CAD build for the part. Positions are in the model's coordinates, mm. A direction names the side the tool comes from. Give positions to 0.01 mm unless a question says otherwise; leave off trailing zeros. Loops run counter-clockwise (first coordinate to the right, second up) from the corner with the lowest first, then second, coordinate; pieces in that order, holes last. Notation, with made-up numbers: M 9.5,-39 L 45.5,-39 A23 cw 45.5,-23 Z; hole C 84.25,30.25 d11. An arc over 180 degrees is marked long. One line per question, with ' | ' between items.
```python
from build123d import *

# Parameters (mm, degrees)
BOSS_EXTRUDE1_DEPTH = 8
CUT_EXTRUDE1_DEPTH  = 1
SKETCH4_W           = 16
SKETCH4_H           = 7
CUT_EXTRUDE2_DEPTH  = 1
SHELL3_START        = 2
SHELL3_DEPTH        = 5.5
SHELL3_START_2      = 0.5
SHELL3_2_DEPTH      = 1.5
SHELL3_START_3      = 1.5
SHELL3_3_OUTLINE_W  = 17
SHELL3_3_OUTLINE_H  = 8
SHELL3_3_DEPTH      = 0.5


# Read off the part's stored shape, not the designer's step: Shell3
with BuildPart() as part:
    # Sketch2 → Boss-Extrude1 (new body)
    with BuildSketch(Plane(origin=(0, 0, 0), x_dir=(1, 0, 0), z_dir=(0, 1, 0))):
        with BuildLine():
            Line((-15, -10), (15, -10))
            ThreePointArc((15, -10), (25, 0), (15, 10))
            Line((15, 10), (-15, 10))
            ThreePointArc((-15, 10), (-25, 0), (-15, -10))
        make_face()
    extrude(amount=BOSS_EXTRUDE1_DEPTH)

    # Sketch3 → Cut-Extrude1 (cut)
    with BuildSketch(Plane.XZ):
        with BuildLine():
            Line((-5, 5), (5, 5))
            ThreePointArc((5, 5), (10, 0), (5, -5))
            Line((5, -5), (-5, -5))
            ThreePointArc((-5, -5), (-10, 0), (-5, 5))
        make_face()
    extrude(amount=-CUT_EXTRUDE1_DEPTH, mode=Mode.SUBTRACT)

    # Sketch4 → Cut-Extrude2 (cut)
    with BuildSketch(Plane.XZ.offset(-1)):
        Rectangle(SKETCH4_W, SKETCH4_H)
    extrude(amount=-CUT_EXTRUDE2_DEPTH, mode=Mode.SUBTRACT)

    # Shell3 outline → Shell3 (cut)
    with BuildSketch(Plane(origin=(0, 0, 0), x_dir=(1, 0, 0), z_dir=(0, 1, 0)).offset(SHELL3_START)):
        with BuildLine():
            Line((15, 9.5), (15, 10))
            Line((15, 10), (-15, 10))
            Line((-15, 10), (-15, 9.5))
            ThreePointArc((-15, 9.5), (-24.5, 0), (-15, -9.5))
            Line((-15, -9.5), (15, -9.5))
            ThreePointArc((15, -9.5), (24.5, 0), (15, 9.5))
        make_face()
    extrude(amount=SHELL3_DEPTH, mode=Mode.SUBTRACT)

    # Shell3 2 outline → Shell3 2 (cut)
    with BuildSketch(Plane(origin=(0, 0, 0), x_dir=(1, 0, 0), z_dir=(0, 1, 0)).offset(SHELL3_START_2)):
        with BuildLine():
            Line((15, 9.5), (15, 10))
            Line((15, 10), (-15, 10))
            Line((-15, 10), (-15, 9.5))
            ThreePointArc((-15, 9.5), (-24.5, 0), (-15, -9.5))
            Line((-15, -9.5), (15, -9.5))
            ThreePointArc((15, -9.5), (24.5, 0), (15, 9.5))
        make_face()
        with BuildLine():
            Line((5, -5.5), (-5, -5.5))
            ThreePointArc((-5, -5.5), (-10.5, 0), (-5, 5.5))
            Line((-5, 5.5), (5, 5.5))
            ThreePointArc((5, 5.5), (10.5, 0), (5, -5.5))
        make_face(mode=Mode.SUBTRACT)
    extrude(amount=SHELL3_2_DEPTH, mode=Mode.SUBTRACT)

    # Shell3 3 outline → Shell3 3 (cut)
    with BuildSketch(Plane(origin=(0, 0, 0), x_dir=(1, 0, 0), z_dir=(0, 1, 0)).offset(SHELL3_START_3)):
        with BuildLine():
            ThreePointArc((-5, 5.5), (-10.5, 0), (-5, -5.5))
            Line((-5, -5.5), (5, -5.5))
            ThreePointArc((5, -5.5), (10.5, 0), (5, 5.5))
            Line((5, 5.5), (-5, 5.5))
        make_face()
        Rectangle(SHELL3_3_OUTLINE_W, SHELL3_3_OUTLINE_H, mode=Mode.SUBTRACT)
    extrude(amount=SHELL3_3_DEPTH, mode=Mode.SUBTRACT)


solid = part.part
```
Item 1: Saw through at D-D on y = 5.25. Give the cut face in (x, z), and give its area (3 significant figures).
Conclusion:
outline: M -15,-10 L -15,-9.5 A9.5 cw -15,9.5 L 15,9.5 A9.5 cw 15,-9.5 L 15,-10 A10 ccw 15,10 L -15,10 A10 ccw Z | area: 45.6 mm²
Item 2: Mould opens along Y. For faces 5 (the flat face through (0, 1, 5.5)), 6 (the flat face through (0, 1, -4)), 7 (the flat face through (0.1, 0.5, -5)) say: pulls with the +Y half, pulls with the -Y half, needs draft (parallel to the pull), parting line crosses it, or undercut.
Conclusion:
face 5: undercut | face 6: pulls with the -Y half | face 7: needs draft
Item 3: Saw through at C-C on z = 0. Give the cut face in (x, y).
Conclusion:
outline: M -25,0 L -10,0 L -10,1 L -8,1 L -8,2 L -8.5,2 L -8.5,1.5 L -10.5,1.5 L -10.5,0.5 L -24.5,0.5 L -24.5,7.5 L 24.5,7.5 L 24.5,0.5 L 10.5,0.5 L 10.5,1.5 L 8.5,1.5 L 8.5,2 L 8,2 L 8,1 L 10,1 L 10,0 L 25,0 L 25,8 L -25,8 Z
Item 4: Drop flat-ended pins along their axis: P1, Ø8, axis at x = 3.5, z = 0, coming from the -Y side; P2, Ø2, axis at y = 3, z = -2, coming from the -X side; P3, Ø0.6, axis at y = 2, z = 1, coming from the +X side. Give the stop position or say it passes through.
Conclusion:
P1: y = 1 | P2: x = -24.95 | P3: x = 24.98
Item 5: Saw through at A-A on x = -19. Give the cut face in (y, z), and give its area (3 significant figures).
Conclusion:
outline: M 0,-9.17 L 8,-9.17 L 8,9.17 L 0,9.17 Z; hole M 0.5,-8.62 L 7.5,-8.62 L 7.5,8.62 L 0.5,8.62 Z | area: 26.0 mm²
Item 6: Saw through at B-B on z = 6.25. Give the cut face in (x, y).
Conclusion:
outline: M -22.81,0 L 22.81,0 L 22.81,8 L -22.81,8 Z; hole M -22.15,0.5 L 22.15,0.5 L 22.15,7.5 L -22.15,7.5 Z
Item 7: 3-axis set-ups, long thin cutter, end or side, ignore diameter. For faces 1 (the flat face through (8, 1.5, 0)), 2 (the flat face through (0, 2, 3.8)), 3 (the cylindrical face through (24.498, 3.951, 0.209)), 4 (the flat face through (0, 4, 10)): which of +Z, -Z, +X, -X, +Y, -Y reach the whole face in a straight line?
Conclusion:
face 1: -Y | face 2: -Z | face 3: none | face 4: +Z, +X, -X, +Y, -Y
Item 8: Drill centre lines: line 1 along Y through (x, z) = (-8, -6.5); line 2 along Y through (x, z) = (-6, 4.5); line 3 along X through (y, z) = (6.75, -4). Where is each one in solid material? Low to high. Write a range as [from, to].
Conclusion:
line 1: [0, 0.5], [7.5, 8] | line 2: [1, 1.5], [7.5, 8] | line 3: [-24.17, -23.62], [23.62, 24.17]
